Part model, mm, in its own coordinate system. Face numbers are marked on the shaded views. A direction names the side the tool comes from. Round coordinates to 2 decimals unless told otherwise and drop trailing zeros. Write each loop counter-clockwise with the first axis right and the second up, starting at its lowest first coordinate (ties: lowest second). Pieces come first, ordered by that corner, then holes.
1) Saw through at C-C on x = 7.5. Write the cut outline in (y, z) (3 decimals).
2) Drill centre lines: L1, parallel to X at y = 0, z = 60 (3 decimals); L2, parallel to Y at x = 2.5, z = 9; L3, parallel to Y at x = -0.5, z = 9. Where is each one in solid material? Low to high.
3) Flat gauge pins, fed straight in: pin 1 (5.5 mm diameter, centred on x = 1, y = -12.5, fed in from +Z); pin 2 (9 mm diameter, centred on x = -14.5, z = 75.5, fed in from -Y); pin 3 (2.5 mm diameter, centred on y = -14.5, z = 77, fed in from +X). Where does each tip first touch, or does it go through?
4) Saw through at A-A on y = 0. Write the cut outline in (x, z) (3 decimals), and give its area (3 significant figures).
5) Which spindle directions (+Z, -Z, +X, -X, +Y, -Y) get a long thin tool onto all of the face, cutting with end or side? Do the marked faces 1, 2, 3 and 4. Say none if no direction does.
```python
from build123d import *

# Parameters (mm, degrees)
F0_R     = 22.225
F1_DEPTH = 82.55
F3_DEPTH = 9.525
F4_SIZE  = 1.27
F5_R     = 22.225
F5_W     = 25.4
F5_H     = 25.4
F6_DEPTH = 12.7
F7_R     = 1.27
F8_R     = 6.35
F9_DEPTH = 82.551


with BuildPart() as f1:
    # F0 (on Top) → F1 (new body)
    with BuildSketch(Plane.XY):
        Circle(F0_R)
    extrude(amount=F1_DEPTH)

    # F2 (on face) → F3 (cut)
    with BuildSketch(Plane.XY.offset(82.55)):
        with BuildLine():
            ThreePointArc((2.54, 22.0793800864), (0, 22.225), (-2.54, 22.0793800864))
            Line((-2.54, 22.0793800864), (-2.54, 2.54))
            Line((-2.54, 2.54), (-22.0793800864, 2.54))
            ThreePointArc((-22.0793800864, 2.54), (-22.225, 0), (-22.0793800864, -2.54))
            Line((-22.0793800864, -2.54), (-2.54, -2.54))
            Line((-2.54, -2.54), (-2.54, -22.0793800864))
            ThreePointArc((-2.54, -22.0793800864), (0, -22.225), (2.54, -22.0793800864))
            Line((2.54, -22.0793800864), (2.54, -2.54))
            Line((2.54, -2.54), (22.0793800864, -2.54))
            ThreePointArc((22.0793800864, -2.54), (22.1885651566, -1.2720854098), (22.225, 0))
            ThreePointArc((22.225, 0), (22.1885651566, 1.2720854098), (22.0793800864, 2.54))
            Line((22.0793800864, 2.54), (2.54, 2.54))
            Line((2.54, 2.54), (2.54, 22.0793800864))
        make_face()
    extrude(amount=-F3_DEPTH, mode=Mode.SUBTRACT)

    # F4
    f4_edges = [f1.edges().sort_by_distance(p)[0] for p in [
        (-12.30969, 2.54, 82.55),
        (-2.54, 12.30969, 82.55),
        (2.54, 12.30969, 82.55),
        (12.30969, 2.54, 82.55),
        (12.30969, -2.54, 82.55),
        (2.54, -12.30969, 82.55),
        (-2.54, -12.30969, 82.55),
        (-12.30969, -2.54, 82.55),
    ]]
    chamfer(f4_edges, length=F4_SIZE)

    # F5 (on face) → F6 (cut)
    with BuildSketch(Plane(origin=(0, 0, 0), x_dir=(1, 0, 0), z_dir=(0, 0, -1))):
        Circle(F5_R)
        Rectangle(F5_W, F5_H, mode=Mode.SUBTRACT)
    extrude(amount=-F6_DEPTH, mode=Mode.SUBTRACT)

    # F7
    f7_edges = [f1.edges().sort_by_distance(p)[0] for p in [
        (0, 12.7, 12.7),
        (12.7, 0, 12.7),
        (-12.7, 0, 12.7),
        (0, -12.7, 12.7),
    ]]
    fillet(f7_edges, radius=F7_R)

    # F8 (on face) → F9 (cut, through all)
    with BuildSketch(Plane(origin=(0, 0, 0), x_dir=(1, 0, 0), z_dir=(0, 0, -1))):
        Circle(F8_R)
    extrude(amount=-F9_DEPTH, mode=Mode.SUBTRACT)


solid = f1.part
```
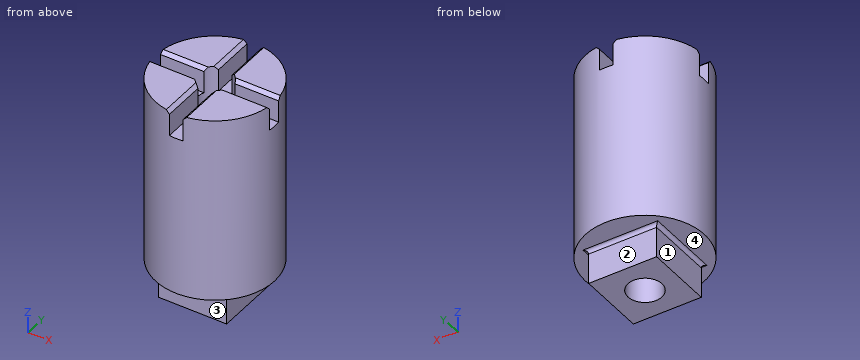
Completed:
1. outline: (-20.921, 12.7) - (-13.97, 12.7) arc R1.27 cw to (-12.7, 11.43) - (-12.7, 0) - (12.7, 0) - (12.7, 11.43) arc R1.27 cw to (13.97, 12.7) - (20.921, 12.7) - (20.921, 82.55) - (3.81, 82.55) - (2.54, 81.28) - (2.54, 73.025) - (-2.54, 73.025) - (-2.54, 81.28) - (-3.81, 82.55) - (-20.921, 82.55) - close
2. L1: x = -22.225 to -6.35, 6.35 to 22.225
2. L2: y = -12.7 to -5.84, 5.84 to 12.7
2. L3: y = -12.7 to -6.33, 6.33 to 12.7
3. pin 1: stops at z = 82.49
3. pin 2: stops at y = -19.85
3. pin 3: stops at x = 17.84
4. outline: (-22.225, 12.7) - (-13.97, 12.7) arc R1.27 cw to (-12.7, 11.43) - (-12.7, 0) - (-6.35, 0) - (-6.35, 73.025) - (-22.225, 73.025) - close; (6.35, 0) - (12.7, 0) - (12.7, 11.43) arc R1.27 cw to (13.97, 12.7) - (22.225, 12.7) - (22.225, 73.025) - (6.35, 73.025) - close
4. area: 2,080 mm2
5. face 1: -Z, -X, +Y, -Y
5. face 2: -Z, +X, -X, +Y
5. face 3: -Z, +X, -X, -Y
5. face 4: -Z
